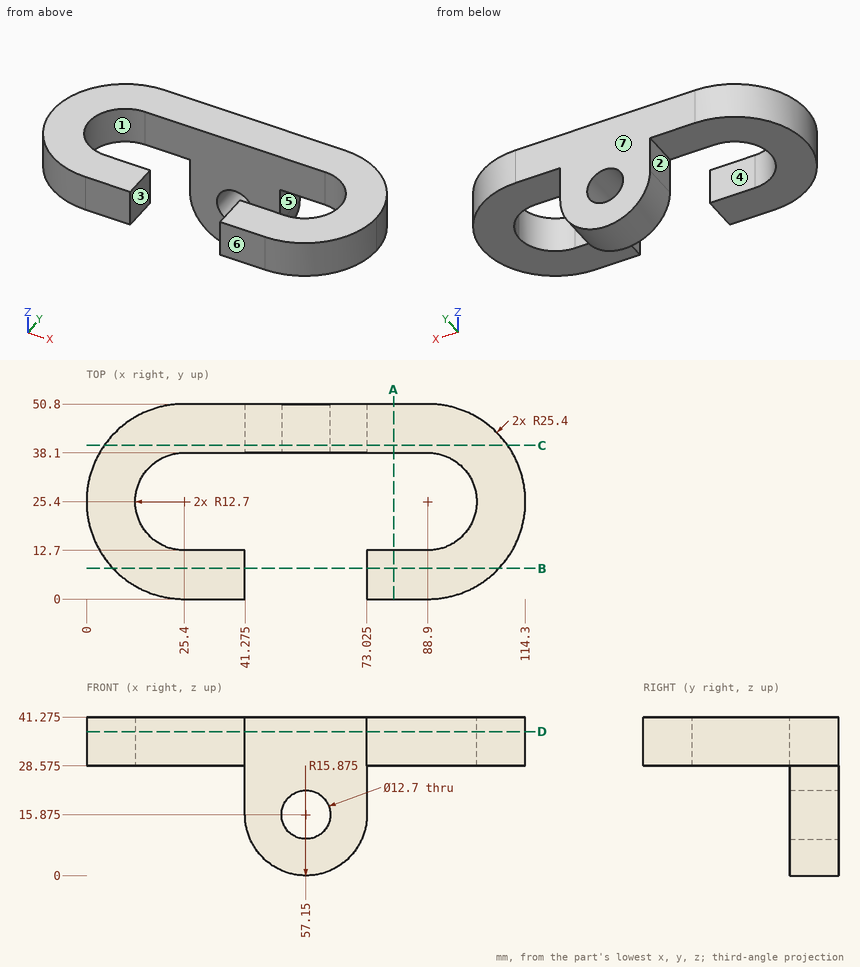
Geometry: see drawing. Coordinates: mm, zero at the bounding-box minimum. A direction names the side the tool comes from. Round coordinates to 2 decimals unless told otherwise and drop trailing zeros. Loops run counter-clockwise (first coordinate to the right, second up) from the corner with the lowest first, then second, coordinate; pieces in that order, holes last.
(1) Section query D-D (z = 37.5). Output: boundary loops of the cut face in (x, y) (3 decimals).
From the geometry:
outline: (25.4, 0) - (41.275, 0) - (41.275, 12.7) - (25.4, 12.7) arc R12.7 cw to (25.4, 38.1) - (88.9, 38.1) arc R12.7 cw to (88.9, 12.7) - (73.025, 12.7) - (73.025, 0) - (88.9, 0) arc R25.4 ccw to (114.3, 25.4) arc R25.4 ccw to (88.9, 50.8) - (25.4, 50.8) arc R25.4 ccw to start
(2) Section query B-B (y = 8). Output: boundary loops of the cut face in (x, z) (3 decimals).
From the geometry:
outline: (6.896, 28.575) - (41.275, 28.575) - (41.275, 41.275) - (6.896, 41.275) - close; (73.025, 28.575) - (107.404, 28.575) - (107.404, 41.275) - (73.025, 41.275) - close
(3) Section query A-A (x = 80). Output: boundary loops of the cut face in (y, z) (3 decimals), and give its area (3 significant figures).
From the geometry:
outline: (0, 28.575) - (12.7, 28.575) - (12.7, 41.275) - (0, 41.275) - close; (38.1, 28.575) - (50.8, 28.575) - (50.8, 41.275) - (38.1, 41.275) - close
area: 323 mm2
(4) Contact query for flat-ended pins moving along their axis: pin 1 Ø4 at (y, z) = (4.5, 32) entering from +X; pin 2 Ø12 at (y, z) = (22.5, 22) entering from +X; pin 3 Ø10 at (y, z) = (42.5, 24) entering from -X; pin 4 Ø12.5 at (x, y) = (98.5, 21.5) entering from -Z (3 decimals). Output: stop coordinate, or through.
From the geometry:
pin 1: stops at x = 105.87
pin 2: passes through
pin 3: stops at x = 4.96
pin 4: stops at z = 28.575
(5) Material intervals for probe 1 along Z at (x, y) = (57, 44) (3 decimals); probe 2 along Y at (x, z) = (78, 29); probe 3 along Z at (x, y) = (18.5, 37) (3 decimals), sorted ascending.
From the geometry:
probe 1: z = 0.001 to 9.527, 22.223 to 41.275
probe 2: y = 0 to 12.7, 38.1 to 50.8
probe 3: z = 28.575 to 41.275
(6) Access query for the marked faces 1, 2 and 3. Directions: +Z, -Z, +X, -X, +Y, -Y. A direction counts if a zero-diameter tool reaches every point of the face in a straight line with its end or side. Return the directions, or none.
From the geometry:
face 1: +Z, -Z
face 2: -Z, -X, +Y, -Y
face 3: +Z, -Z, -Y
(7) Pull-direction query (Y, two-part tool) for the marked faces 4, 5, 6 and 7; classes: +Y half, -Y half, draft (parallel to the pull), parting line (faces both ways), or undercut.
From the geometry:
face 4: undercut
face 5: draft
face 6: -Y half
face 7: +Y half
(8) Section query C-C (y = 40). Output: boundary loops of the cut face in (x, z) (3 decimals).
From the geometry:
outline: (4.615, 28.575) - (41.275, 28.575) - (41.275, 15.875) arc R15.875 ccw to (73.025, 15.875) - (73.025, 28.575) - (109.685, 28.575) - (109.685, 41.275) - (4.615, 41.275) - close; hole circle Ø12.7 at (57.15, 15.875)
